```python
from build123d import *

# Parameters (mm, degrees)
SKETCH_1_W                  = 80
SKETCH_1_H                  = 145
SKETCH_1_R                  = 19.05
EXTRUDE_1_DEPTH             = 10
CUT_EXTRUDE_1_DEPTH         = 6
HOLE_WIZARD_M51_D           = 4.2
HOLE_WIZARD_M51_DEPTH       = 14
HOLE_WIZARD_M51_CSINK_D     = 5.05
HOLE_WIZARD_M51_CSINK_ANGLE = 120
HOLE_WIZARD_M51_TIP         = 1.2618073
SKETCH_5_R                  = 3
CUT_EXTRUDE_2_DEPTH         = 7
HOLE_WIZARD_M41_D           = 4.5
HOLE_WIZARD_M41_CSINK_D     = 9.18
HOLE_WIZARD_M41_CSINK_ANGLE = 90


with BuildPart() as part:
    # Эскиз1 → Бобышка-Вытянуть1 (new body)
    with BuildSketch(Plane.XY):
        with Locations((40, 72.5)):
            Rectangle(SKETCH_1_W, SKETCH_1_H)
        with Locations((40, 116.8)):
            Circle(SKETCH_1_R, mode=Mode.SUBTRACT)
        with BuildLine():
            Line((18.25, 60), (18.25, 50))
            ThreePointArc((18.25, 50), (15, 46.75), (11.75, 50))
            Line((11.75, 50), (11.75, 60))
            ThreePointArc((11.75, 60), (15, 63.25), (18.25, 60))
        make_face(mode=Mode.SUBTRACT)
        with BuildLine():
            Line((18.25, 20), (18.25, 10))
            ThreePointArc((18.25, 10), (15, 6.75), (11.75, 10))
            Line((11.75, 10), (11.75, 20))
            ThreePointArc((11.75, 20), (15, 23.25), (18.25, 20))
        make_face(mode=Mode.SUBTRACT)
        with BuildLine():
            Line((61.75, 20), (61.75, 10))
            ThreePointArc((61.75, 10), (65, 6.75), (68.25, 10))
            Line((68.25, 10), (68.25, 20))
            ThreePointArc((68.25, 20), (65, 23.25), (61.75, 20))
        make_face(mode=Mode.SUBTRACT)
        with BuildLine():
            Line((61.75, 60), (61.75, 50))
            ThreePointArc((61.75, 50), (65, 46.75), (68.25, 50))
            Line((68.25, 50), (68.25, 60))
            ThreePointArc((68.25, 60), (65, 63.25), (61.75, 60))
        make_face(mode=Mode.SUBTRACT)
    extrude(amount=EXTRUDE_1_DEPTH)

    # Эскиз4 → Вырез-Вытянуть1 (cut)
    with BuildSketch(Plane(origin=(0, 0, 0), x_dir=(-1, 0, 0), z_dir=(0, 0, -1))):
        with BuildLine():
            Line((-68.5, 145), (-11.5, 145))
            Line((-11.5, 145), (-11.5, 90.5))
            ThreePointArc((-11.5, 90.5), (-12.232233047, 88.732233047), (-14, 88))
            Line((-14, 88), (-66, 88))
            ThreePointArc((-66, 88), (-67.767766953, 88.732233047), (-68.5, 90.5))
            Line((-68.5, 90.5), (-68.5, 145))
        make_face()
    extrude(amount=-CUT_EXTRUDE_1_DEPTH, mode=Mode.SUBTRACT)

    # Отверстие обработанное метчиком M51
    with Locations(Plane(origin=(24.344692429, -10.713064845, 6), x_dir=(-1, 0, 0), z_dir=(0, 0, -1))):
        with Locations((7.914692429, 103.943064845), (7.914692429, 151.083064845), (-39.225307571, 151.083064845), (-39.225307571, 103.943064845)):
            CounterSinkHole(HOLE_WIZARD_M51_D / 2, HOLE_WIZARD_M51_CSINK_D / 2, depth=HOLE_WIZARD_M51_DEPTH, counter_sink_angle=HOLE_WIZARD_M51_CSINK_ANGLE)
            with Locations((0, 0, -(HOLE_WIZARD_M51_DEPTH + HOLE_WIZARD_M51_TIP / 2))):  # 118° drill point
                Cone(0, HOLE_WIZARD_M51_D / 2, HOLE_WIZARD_M51_TIP, mode=Mode.SUBTRACT)

    # Эскиз5 → Вырез-Вытянуть2 (cut)
    with BuildSketch(Plane.XY.offset(10)):
        with Locations((22, 80)):
            Circle(SKETCH_5_R)
        with Locations((58, 80)):
            Circle(SKETCH_5_R)
    extrude(amount=-CUT_EXTRUDE_2_DEPTH, mode=Mode.SUBTRACT)

    # Зенковка для винта с потайной головкой и внутренним шестигранником M41 (through all)
    with Locations(Plane(origin=(0, 0, 0), x_dir=(-1, 0, 0), z_dir=(0, 0, -1))):
        with Locations((-22, 80), (-58, 80)):
            CounterSinkHole(HOLE_WIZARD_M41_D / 2, HOLE_WIZARD_M41_CSINK_D / 2, counter_sink_angle=HOLE_WIZARD_M41_CSINK_ANGLE)


solid = part.part
```
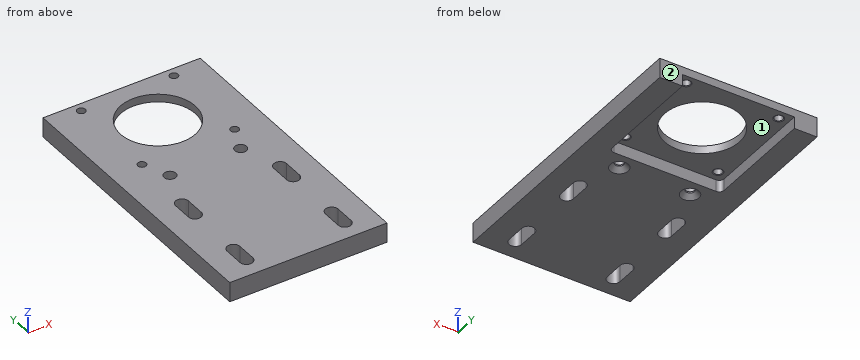
Geometry: final body of the model. Coordinates: model frame, mm. Face numbers are marked on the shaded views. A direction names the side the tool comes from. Coordinates: 2 decimals unless noted, no trailing zeros. Order: outer loops, then holes, each group sorted by start corner. A loop starts at its lowest first (then second) coordinate and runs counter-clockwise, first axis right, second up. Notation, with made-up numbers: (78.5, 14.25) - (90.5, 14.25) arc R22 cw to (90.5, 30.25) - close; hole circle Ø8 at (40, -16.75). An arc over 180 degrees is marked (long way). Write each question's results on one line, items separated by ' | '.
(1) First-contact query: pin 1 Ø3.5 at (x, y) = (16.43, 140.37) entering from -Z; pin 2 Ø5.5 at (x, y) = (63.57, 93.23) entering from -Z; pin 3 Ø5.5 at (x, y) = (58, 80) entering from -Z. Flat tips, straight axial feed; report the tip coordinate or a pass-through.
Values found:
pin 1: passes through | pin 2: stops at z = 6 | pin 3: stops at z = 1.84
(2) Section query C-C, the plane x = 28.5. Return the cut outline in (y, z).
Values found:
outline: (0, 0) - (88, 0) - (88, 6) - (101.61, 6) - (101.61, 10) - (0, 10) - close; (131.99, 6) - (145, 6) - (145, 10) - (131.99, 10) - close
(3) Section query A-A, the plane y = 52.5. Return the cut outline in (x, z).
Values found:
outline: (0, 0) - (11.75, 0) - (11.75, 10) - (0, 10) - close; (18.25, 0) - (61.75, 0) - (61.75, 10) - (18.25, 10) - close; (68.25, 0) - (80, 0) - (80, 10) - (68.25, 10) - close
(4) Line query: line 1 (X direction, y = 93.23, z = 7.5); line 2 (X direction, y = 50, z = 8.5); line 3 (Y direction, x = 58, z = 2.5). Output: solid intervals per line, ascending. Write a range as [from, to].
Values found:
line 1: x = [0, 14.33], [18.53, 61.47], [65.67, 80] | line 2: x = [0, 11.75], [18.25, 61.75], [68.25, 80] | line 3: y = [0, 77.75], [82.25, 88]
(5) Set-up query: the marked faces 1 and 2. Return all of +Z, -Z, +X, -X, +Y, -Y with unobstructed straight access to the full face (end or side cutting, diameter ignored); none if empty.
Values found:
face 1: -Z, +Y | face 2: +Z, -Z, +X, -X, +Y
(6) Section query B-B, the plane z = 7.75. Count the separate pieces of the cut face and the enclosed holes in it, plus the area to 3 significant figures.
Values found:
separate pieces: 1 | enclosed holes: 11 | area: 9,960 mm²
